Read the model definition and answer for the solid it produces. Units are mm, in the model's axes. Give positions to 0.01 mm unless a question says otherwise; leave off trailing zeros. Order: outer loops, then holes, each group sorted by start corner. A loop starts at its lowest first (then second) coordinate and runs counter-clockwise, first axis right, second up. Notation, with made-up numbers: M -22.5,-16 L -10.5,-16 A10 ccw -10.5,-10 Z; hole C 71.5,-7 d4. An arc over 180 degrees is marked long. One line per item, written item: value. Start each with the question number.
from build123d import *

# Parameters (mm, degrees)
SKETCH1_W           = 247.65
SKETCH1_H           = 76.3524
SKETCH1_R           = 4.25
SKETCH1_R_2         = 2.25
SKETCH1_R_3         = 3.175
SKETCH1_W_2         = 2
SKETCH1_H_2         = 3.2
SKETCH1_W_3         = 1
SKETCH1_H_3         = 2.5
BOSS_EXTRUDE1_DEPTH = 1.6


with BuildPart() as part:
    # Sketch1 → Boss-Extrude1 (new body)
    with BuildSketch(Plane(origin=(0, 0, 0), x_dir=(1, 0, 0), z_dir=(0, 1, 0))):
        with Locations((123.825, 38.1762)):
            Rectangle(SKETCH1_W, SKETCH1_H)
        with Locations(Location((208.518808658, 13.416643134, 0), (0, 0, 270))):  # turned: the seam where the file's is
            Circle(SKETCH1_R, mode=Mode.SUBTRACT)
        with Locations(Location((191.691308658, 13.416643134, 0), (0, 0, 270))):  # turned: the seam where the file's is
            Circle(SKETCH1_R, mode=Mode.SUBTRACT)
        with Locations(Location((164.119003876, 12.968247461, 0), (0, 0, 270))):  # turned: the seam where the file's is
            Circle(SKETCH1_R, mode=Mode.SUBTRACT)
        with Locations(Location((147.291503876, 12.968247461, 0), (0, 0, 270))):  # turned: the seam where the file's is
            Circle(SKETCH1_R, mode=Mode.SUBTRACT)
        with Locations(Location((200.105058658, 33.963274369, 0), (0, 0, 270))):  # turned: the seam where the file's is
            Circle(SKETCH1_R, mode=Mode.SUBTRACT)
        with Locations(Location((155.705253876, 33.49674194, 0), (0, 0, 270))):  # turned: the seam where the file's is
            Circle(SKETCH1_R, mode=Mode.SUBTRACT)
        with Locations(Location((25, 46.3524, 0), (0, 0, 270))):  # turned: the seam where the file's is
            Circle(SKETCH1_R_2, mode=Mode.SUBTRACT)
        with Locations(Location((42.853159836, 37.07576509, 0), (0, 0, 270))):  # turned: the seam where the file's is
            Circle(SKETCH1_R_3, mode=Mode.SUBTRACT)
        with Locations((211.855058658, 33.49674194)):
            Rectangle(SKETCH1_W_2, SKETCH1_H_2, mode=Mode.SUBTRACT)
        with Locations((167.455253876, 33.49674194)):
            Rectangle(SKETCH1_W_2, SKETCH1_H_2, mode=Mode.SUBTRACT)
        with Locations((49.128159836, 37.07576509)):
            Rectangle(SKETCH1_W_3, SKETCH1_H_3, mode=Mode.SUBTRACT)
    extrude(amount=BOSS_EXTRUDE1_DEPTH)


solid = part.part
Q1. This flat-tipped pin is pushed along its axis until it touches: pin 1 (13.5 mm diameter, centred on x = 147.29, z = -12.97, fed in from -Y). Where does it stop, or does it pass through?
Q2. Find section C-C, the plane y = 0.9. State how many separate pieces and enclosed holes the cut face has, then the cut area to 3 significant figures.
Q3. Determine the mould class of faces 1 (the flat face through (122, 0, -39)), 2 (the cylindrical face through (204.37, 0.79, -14.34)) for opening direction Z: released by +Z, released by -Z, zero draft, split by the parting line, or undercut.
Q4. Find section A-A, the plane x = 25. Give the vertices of the cut face in (y, z).
Q5. Find section B-B, the plane z = -15. Give the vertices of the cut face in (x, y).
Q6. Consider probe 1 along Z at (x, y) = (42.5, 1.45); probe 2 along X at (y, z) = (0.6, -11.5); probe 3 along X at (y, z) = (1.3, -36). Determine where each line is inside the solid, lowest interval first.
Evaluation:
1. pin 1: y = 0
2. separate pieces: 1
2. enclosed holes: 11
2. area: 18,500 mm2
3. face 1: zero draft
3. face 2: undercut
4. outline: M 0,-76.35 L 1.6,-76.35 L 1.6,-48.6 L 0,-48.6 Z; M 0,-44.1 L 1.6,-44.1 L 1.6,0 L 0,0 Z
5. outline: M 0,0 L 143.56,0 L 143.56,1.6 L 0,1.6 Z; M 151.02,0 L 160.39,0 L 160.39,1.6 L 151.02,1.6 Z; M 167.85,0 L 187.75,0 L 187.75,1.6 L 167.85,1.6 Z; M 195.64,0 L 204.57,0 L 204.57,1.6 L 195.64,1.6 Z; M 212.46,0 L 247.65,0 L 247.65,1.6 L 212.46,1.6 Z
6. probe 1: -76.35 to -40.23, -33.92 to 0
6. probe 2: 0 to 143.3, 151.28 to 160.13, 168.11 to 187.9, 195.48 to 204.73, 212.31 to 247.65
6. probe 3: 0 to 39.87, 45.84 to 48.63, 49.63 to 152.27, 159.14 to 196.37, 203.84 to 247.65
